Design review of the part built by this model. Coordinates are the model's own, in mm. Give positions to 0.01 mm unless a question says otherwise; leave off trailing zeros. Write each loop counter-clockwise with the first axis right and the second up, starting at its lowest first coordinate (ties: lowest second). Pieces come first, ordered by that corner, then holes. Notation, with made-up numbers: (73, 17.5) -> (112, 17.5) arc R8 cw to (112, 22.5) -> close; hole circle Ø2 at (71, -7.75). An arc over 180 degrees is marked (long way). Answer as a JSON object with one key per item and string values.
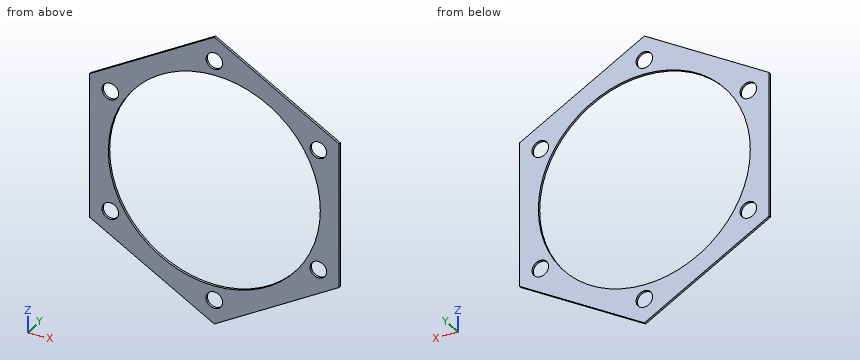
```python
from build123d import *

# Parameters (mm, degrees)
BOSS_EXTRUDE1_DEPTH = 1
SKETCH2_R           = 45
SKETCH2_R_2         = 3.5
CUT_EXTRUDE1_DEPTH  = 81.96501302


with BuildPart() as part:
    # Sketch1 → Boss-Extrude1 (new body)
    with BuildSketch(Plane(origin=(0, 0, 0), x_dir=(1, 0, 0), z_dir=(0, 1, 0))):
        Polygon((0, 61.199128534), (-53, 30.599564267), (-53, -30.599564267), (0, -61.199128534), (53, -30.599564267), (53, 30.599564267), align=None)
    extrude(amount=BOSS_EXTRUDE1_DEPTH)

    # Sketch2 → Cut-Extrude1 (cut, through all)
    with BuildSketch(Plane(origin=(0, 1, 0), x_dir=(1, 0, 0), z_dir=(0, 1, 0))):
        with Locations(Location((0, 0, 0), (0, 0, 270))):
            Circle(SKETCH2_R)
        with Locations(Location((0, 51, 0), (0, 0, 270))):
            Circle(SKETCH2_R_2)
        with Locations(Location((44.167295593, 25.5, 0), (0, 0, 270))):
            Circle(SKETCH2_R_2)
        with Locations(Location((44.167295593, -25.5, 0), (0, 0, 270))):
            Circle(SKETCH2_R_2)
        with Locations(Location((0, -51, 0), (0, 0, 270))):
            Circle(SKETCH2_R_2)
        with Locations(Location((-44.167295593, -25.5, 0), (0, 0, 270))):
            Circle(SKETCH2_R_2)
        with Locations(Location((-44.167295593, 25.5, 0), (0, 0, 270))):
            Circle(SKETCH2_R_2)
    extrude(amount=-CUT_EXTRUDE1_DEPTH, mode=Mode.SUBTRACT)


solid = part.part
```
(1) Clearance check with a flat-ended pin moving along its axis: pin 1 (5.5 mm diameter, centred on x = 44.17, z = -25.5, fed in from +Y). State where the tip first meets the part, or that it passes through.
Here are the results:
{"pin 1": "passes through"}
(2) For line 1 along X through (y, z) = (0.55, 25.5); line 2 along X through (y, z) = (0.45, 0); line 3 along Z through (x, y) = (11.5, 0.95), list the stretches that pass through material, from the lowest coordinate up.
Here are the results:
{"line 1": "x = -53 to -47.67, -40.67 to -37.08, 37.08 to 40.67, 47.67 to 53", "line 2": "x = -53 to -45, 45 to 53", "line 3": "z = -54.56 to -43.51, 43.51 to 54.56"}
(3) We need section A-A, the plane z = 0. State the section outline as (x, y) points.
Here are the results:
{"outline": "(-53, 0) -> (-45, 0) -> (-45, 1) -> (-53, 1) -> close; (45, 0) -> (53, 0) -> (53, 1) -> (45, 1) -> close"}
(4) We need section B-B, the plane x = 37. State the section outline as (y, z) points.
Here are the results:
{"outline": "(0, -39.84) -> (1, -39.84) -> (1, -25.61) -> (0, -25.61) -> close; (0, 25.61) -> (1, 25.61) -> (1, 39.84) -> (0, 39.84) -> close"}
(5) We need section C-C, the plane z = -25.5. State the section outline as (x, y) points, then the cut area to 3 significant figures.
Here are the results:
{"outline": "(-53, 0) -> (-47.67, 0) -> (-47.67, 1) -> (-53, 1) -> close; (-40.67, 0) -> (-37.08, 0) -> (-37.08, 1) -> (-40.67, 1) -> close; (37.08, 0) -> (40.67, 0) -> (40.67, 1) -> (37.08, 1) -> close; (47.67, 0) -> (53, 0) -> (53, 1) -> (47.67, 1) -> close", "area": "17.8 mm²"}
(6) We need section D-D, the plane y = 0.75. State the section outline as (x, z) points, then the cut area to 3 significant figures.
Here are the results:
{"outline": "(-53, -30.6) -> (0, -61.2) -> (53, -30.6) -> (53, 30.6) -> (0, 61.2) -> (-53, 30.6) -> close; hole circle Ø7 at (-44.17, -25.5); hole circle Ø7 at (-44.17, 25.5); hole circle Ø90 at (0, 0); hole circle Ø7 at (0, -51); hole circle Ø7 at (0, 51); hole circle Ø7 at (44.17, -25.5); hole circle Ø7 at (44.17, 25.5)", "area": "3,140 mm²"}
